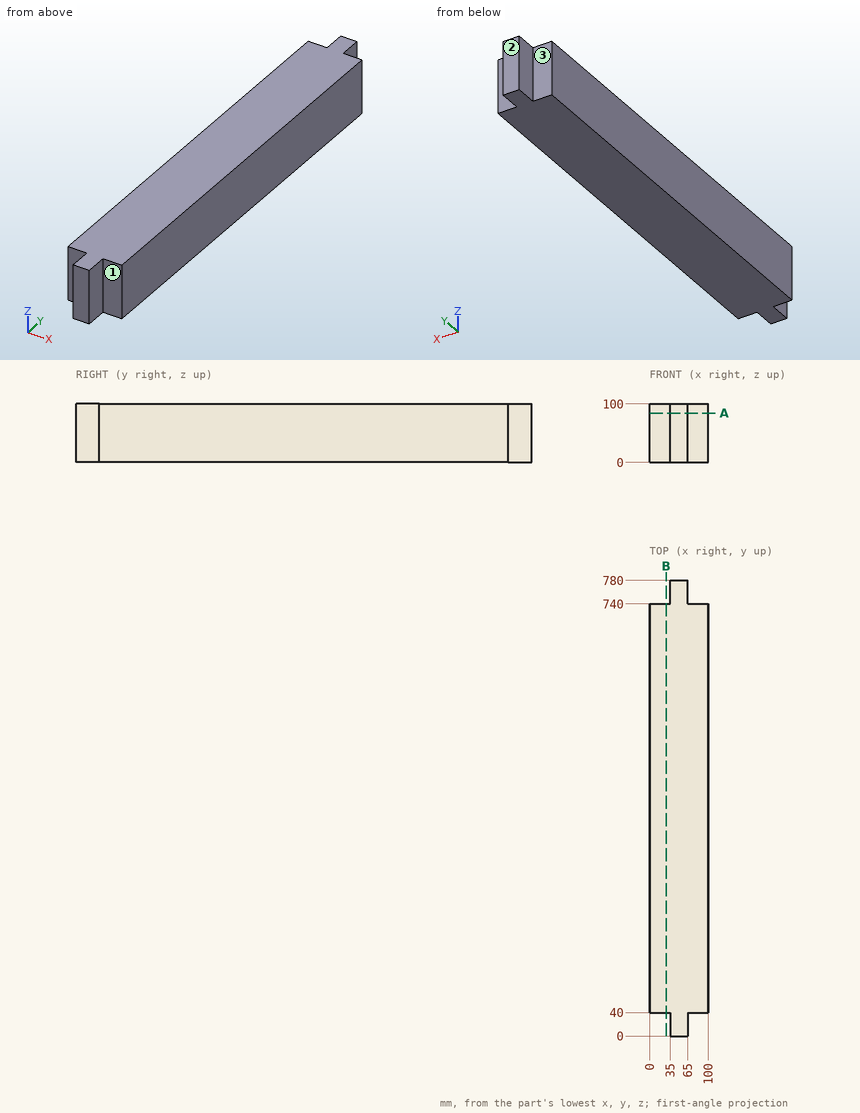
Can you work these out from the drawing? Everything is in mm from the part's minimum corner. A direction names the side the tool comes from. Give positions to 0.01 mm unless a question says otherwise; leave off trailing zeros. Loops run counter-clockwise (first coordinate to the right, second up) from the corner with the lowest first, then second, coordinate; pieces in that order, holes last. Notation, with made-up numbers: (-5.5, -24.75) -> (21.5, -24.75) arc R17 ccw to (21.5, -20.75) -> close; hole circle Ø6 at (47.5, 35). An arc over 180 degrees is marked (long way). Write item = value, one per line.
1) I need wall thicknesses on L1, parallel to Y at x = 94.5, z = 79.5. Which ranges of the line are inside material? Lowest first, please. Write a range as from..to.
Check result:
L1 = 40..740
2) Will these pins go through, and if not, where does the flat tip stop? pin 1 (10.5 mm diameter, centred on x = 24.5, z = 59, fed in from -Y); pin 2 (12 mm diameter, centred on y = 16, z = 55, fed in from +X).
Check result:
pin_1 = 40
pin_2 = 65
3) For the marked faces 1, 2 and 3, which set-ups out of +Z, -Z, +X, -X, +Y, -Y let a thin tool reach every point of the face, with its end or its side?
Check result:
face_1 = +Z, -Z, +X, -Y
face_2 = +Z, -Z, +X, -X, +Y
face_3 = +Z, -Z, -X, +Y
4) Suppose I cut it at B-B on x = 28.5. Write out the boundary of the cut face in (y, z).
Check result:
outline = (40, 0) -> (740, 0) -> (740, 100) -> (40, 100) -> close
5) Suppose I cut it at A-A on z = 84.5. Write out the boundary of the cut face in (x, y).
Check result:
outline = (0, 40) -> (35, 40) -> (35, 0) -> (65, 0) -> (65, 40) -> (100, 40) -> (100, 740) -> (65, 740) -> (65, 780) -> (35, 780) -> (35, 740) -> (0, 740) -> close
